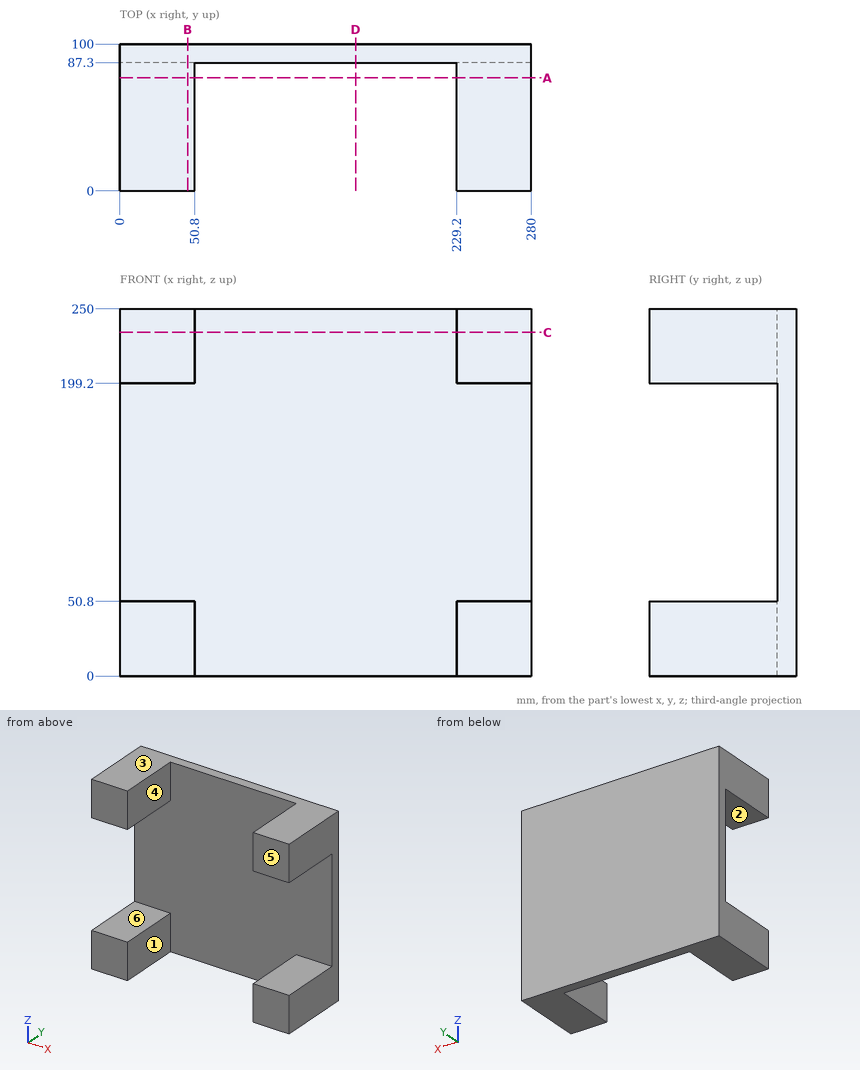
Drawing for the job (mm, zero at the part's lowest x, y, z). A direction names the side the tool comes from. Round coordinates to 2 decimals unless told otherwise and drop trailing zeros. Write each loop counter-clockwise with the first axis right and the second up, starting at its lowest first coordinate (ties: lowest second). Pieces come first, ordered by that corner, then holes. Notation, with made-up numbers: (-32.5, -20.75) - (2.5, -20.75) arc R27 cw to (2.5, 7.25) - close; hole circle Ø7 at (-16.75, 24.25). An arc over 180 degrees is marked (long way). Use CSV: the item, a comma, the result in double quotes.
(1) Pin check, flat tip, straight feed: P1, Ø1.5, axis at x = 133, z = 104.5, coming from the -Y side. Stop position of the tip, or through.
Response:
P1,"y = 87.3"
(2) Band-saw the part on B-B (x = 46). Write the cut outline in (y, z), plus the area to 3 significant figures.
Response:
outline,"(0, 0) - (100, 0) - (100, 250) - (0, 250) - (0, 199.2) - (87.3, 199.2) - (87.3, 50.8) - (0, 50.8) - close"
area,"12,000 mm²"
(3) Band-saw the part on C-C (z = 234). Write the cut outline in (x, y).
Response:
outline,"(0, 0) - (50.8, 0) - (50.8, 87.3) - (229.2, 87.3) - (229.2, 0) - (280, 0) - (280, 100) - (0, 100) - close"
(4) Band-saw the part on D-D (x = 160.5). Write the cut outline in (y, z).
Response:
outline,"(87.3, 0) - (100, 0) - (100, 250) - (87.3, 250) - close"
(5) Mould opens along Z. For the marked faces 1, 2 and 3 say: pulls with the +Z half, pulls with the -Z half, needs draft (parallel to the pull), parting line crosses it, or undercut.
Response:
face 1,"needs draft"
face 2,"undercut"
face 3,"pulls with the +Z half"
(6) 3-axis set-ups, long thin cutter, end or side, ignore diameter. For the marked faces 4, 5 and 6: which of +Z, -Z, +X, -X, +Y, -Y reach the whole face in a straight line?
Response:
face 4,"+Z, -Z, -Y"
face 5,"+Z, -Z, +X, -X, -Y"
face 6,"+X, -X, -Y"
(7) Wall check: line 1 (Z direction, x = 256.5, y = 77.5); line 2 (X direction, y = 85.5, z = 239.5); line 3 (Y direction, x = 135.5, z = 238). Give the ranges that are in metal, low to high.
Response:
line 1,"0 to 50.8, 199.2 to 250"
line 2,"0 to 50.8, 229.2 to 280"
line 3,"87.3 to 100"
(8) Band-saw the part on A-A (y = 77). Write the cut outline in (x, z).
Response:
outline,"(0, 0) - (50.8, 0) - (50.8, 50.8) - (0, 50.8) - close; (0, 199.2) - (50.8, 199.2) - (50.8, 250) - (0, 250) - close; (229.2, 0) - (280, 0) - (280, 50.8) - (229.2, 50.8) - close; (229.2, 199.2) - (280, 199.2) - (280, 250) - (229.2, 250) - close"
